```python
from build123d import *

# Parameters (mm, degrees)
SKETCH2_W               = 18
SKETCH2_H               = 43.5
BOSS_EXTRUDE1_DEPTH     = 25
CUT_EXTRUDE1_DEPTH      = 15
CUT_EXTRUDE1_DEPTH_BACK = 6.951267747
CUT_EXTRUDE2_START      = 0.4
CUT_EXTRUDE2_DEPTH      = 3.3
SKETCH5_W               = 15
SKETCH5_H               = 43.5
BOSS_EXTRUDE2_DEPTH     = 120
SKETCH6_W               = 2.2
SKETCH6_H               = 14.9
CUT_EXTRUDE3_DEPTH      = 2
CUT_EXTRUDE4_START      = -43.5
SKETCH6_3_W             = 2.2
SKETCH6_3_H             = 14.9
CUT_EXTRUDE4_DEPTH      = 2
CUT_EXTRUDE5_DEPTH      = 44.5
SKETCH8_W               = 37.1
SKETCH8_H               = 38
CUT_EXTRUDE6_DEPTH      = 16
FILLET1_R               = 10


with BuildPart() as part:
    # Sketch2 → Boss-Extrude1 (new body)
    with BuildSketch(Plane(origin=(0, 0, 0), x_dir=(1, 0, 0), z_dir=(0, 1, 0))):
        with BuildLine():
            Line((-9, 0), (-9, 21.75))
            Line((-9, 21.75), (-14.951267747, 10.950365309))
            ThreePointArc((-14.951267747, 10.950365309), (-10.583942354, 6.231534486), (-9, 0))
        make_face()
        with BuildLine():
            Line((-9, -21.75), (-9, 0))
            ThreePointArc((-9, 0), (-10.583942354, -6.231534486), (-14.951267747, -10.950365309))
            Line((-14.951267747, -10.950365309), (-9, -21.75))
        make_face()
        Rectangle(SKETCH2_W, SKETCH2_H)
    extrude(amount=BOSS_EXTRUDE1_DEPTH)

    # Sketch3 → Cut-Extrude1 (cut, two sides)
    with BuildSketch(Plane(origin=(-9, 0, 0), x_dir=(0, 0, -1), z_dir=(1, 0, 0))) as cut_extrude1_sk:
        Polygon((-5.15, 25), (5.15, 25), (7.15, 21.535898385), (-7.15, 21.535898385), align=None)
    extrude(amount=CUT_EXTRUDE1_DEPTH, mode=Mode.SUBTRACT)
    extrude(cut_extrude1_sk.sketch, amount=-CUT_EXTRUDE1_DEPTH_BACK, mode=Mode.SUBTRACT)

    # Sketch4 → Cut-Extrude2 (cut)
    with BuildSketch(Plane(origin=(-9, 0, 0), x_dir=(0, 0, -1), z_dir=(1, 0, 0)).offset(CUT_EXTRUDE2_START)):
        with BuildLine():
            Line((3.15, 29.404082691), (3.15, 4.535898385))
            ThreePointArc((3.15, 4.535898385), (0, 1.385898385), (-3.15, 4.535898385))
            Line((-3.15, 4.535898385), (-3.15, 29.404082691))
            ThreePointArc((-3.15, 29.404082691), (0, 32.554082691), (3.15, 29.404082691))
        make_face()
    extrude(amount=CUT_EXTRUDE2_DEPTH, mode=Mode.SUBTRACT)

    # Sketch5 → Boss-Extrude2 (add)
    with BuildSketch(Plane.XZ):
        with Locations((1.5, 0)):
            Rectangle(SKETCH5_W, SKETCH5_H)
    extrude(amount=BOSS_EXTRUDE2_DEPTH)

    # Sketch6 → Cut-Extrude3 (cut)
    with BuildSketch(Plane.XY.offset(21.75)):
        Polygon((-3.1, -105.1), (0.4, -105.1), (2.6, -105.1), (6.1, -105.1), (6.1, -100.9), (-3.1, -100.9), align=None)
        with Locations((1.5, -112.55)):
            Rectangle(SKETCH6_W, SKETCH6_H)
    extrude(amount=-CUT_EXTRUDE3_DEPTH, mode=Mode.SUBTRACT)

    # Sketch6<3> → Cut-Extrude4 (cut)
    with BuildSketch(Plane.XY.offset(21.75).offset(CUT_EXTRUDE4_START)):
        Polygon((-3.1, -105.1), (0.4, -105.1), (2.6, -105.1), (6.1, -105.1), (6.1, -100.9), (-3.1, -100.9), align=None)
        with Locations((1.5, -112.55)):
            Rectangle(SKETCH6_3_W, SKETCH6_3_H)
    extrude(amount=CUT_EXTRUDE4_DEPTH, mode=Mode.SUBTRACT)

    # Sketch7 → Cut-Extrude5 (cut, through all)
    with BuildSketch(Plane.XY.offset(21.75)):
        Polygon((9, -116.358920801), (3.8, -120), (9, -120), align=None)
    extrude(amount=-CUT_EXTRUDE5_DEPTH, mode=Mode.SUBTRACT)

    # Sketch8 → Cut-Extrude6 (cut, through all)
    with BuildSketch(Plane.ZY.offset(6)):
        with Locations((0, -120)):
            Rectangle(SKETCH8_W, SKETCH8_H)
    extrude(amount=-CUT_EXTRUDE6_DEPTH, mode=Mode.SUBTRACT)

    # Fillet1
    fillet1_edges = [part.edges().sort_by_distance(p)[0] for p in [
        (1.5, -101, 18.55),
        (1.5, -101, -18.55),
    ]]
    fillet(fillet1_edges, radius=FILLET1_R)


solid = part.part
```
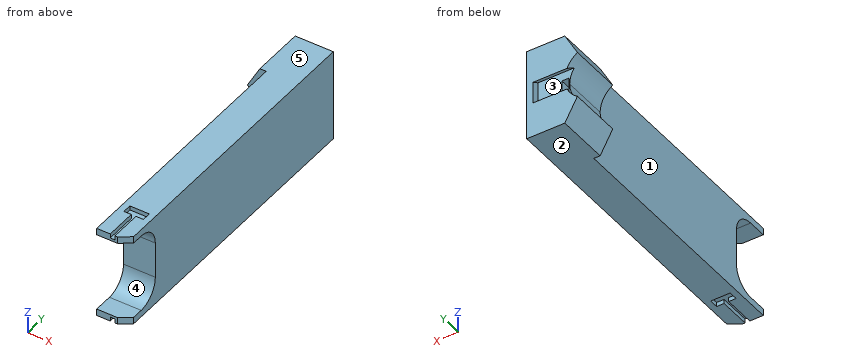
Can you work these out from the model? Positions are in its coordinate system, mm. Face numbers are marked on the shaded views. A direction names the side the tool comes from. Round coordinates to 2 decimals unless told otherwise and drop trailing zeros. Loops run counter-clockwise (first coordinate to the right, second up) from the corner with the lowest first, then second, coordinate; pieces in that order, holes last. Notation, with made-up numbers: (26, 63) -> (31, 63) arc R7 cw to (31, 67) -> close; hole circle Ø4 at (6, -38). An arc over 180 degrees is marked (long way). One line per item, written item: value. Start each with the question number.
1. For the marked faces 4 and 5, which set-ups out of +Z, -Z, +X, -X, +Y, -Y let a thin tool reach every point of the face, with its end or its side?
2. For pin 1 (22 mm diameter, centred on y = -57.5, z = -1, fed in from -X); pin 2 (4.5 mm diameter, centred on x = -9.5, z = 6, fed in from -Y); pin 3 (4 mm diameter, centred on x = 1, z = 0, fed in from -Y), each with a flat end and sliding along its axis, tell me the tip position at first contact or that it passes through.
3. If we section it at A-A, the plane y = 13.5: Write out the boundary of the cut face in (x, z), then the cut area to 3 significant figures.
4. If I drill on probe 1 along X at (y, z) = (-62.5, -9); probe 2 along Y at (x, z) = (-8.75, 10.5); probe 3 along Y at (x, z) = (3.5, 3), over which ranges is the centre line in solid material (lowest first)?
5. If we mould it in two halves opening along Z, with no side actions, what happens to the marked faces 1, 2 and 3? For each: pulls with the +Z half, pulls with the -Z half, needs draft (parallel to the pull), parting line crosses it, or undercut.
6. If we section it at B-B, the plane y = -66: Write out the boundary of the cut face in (x, z), then the cut area to 4 significant figures.
Calculated:
1. face 4: +X, -X, -Y
1. face 5: +Z, +X, -X, +Y, -Y
2. pin 1: stops at x = -6
2. pin 2: stops at y = 0
2. pin 3: stops at y = -101
3. outline: (-14.95, -10.95) -> (-9, -21.75) -> (9, -21.75) -> (9, 21.75) -> (-9, 21.75) -> (-14.95, 10.95) arc R13.05 cw to start; hole (-8.6, -3.15) -> (-5.3, -3.15) -> (-5.3, 3.15) -> (-8.6, 3.15) -> close
3. area: 865 mm²
4. probe 1: x = -6 to 9
4. probe 2: y = 0 to 25
4. probe 3: y = -101 to 21.54
5. face 1: needs draft
5. face 2: pulls with the -Z half
5. face 3: undercut
6. outline: (-6, -21.75) -> (9, -21.75) -> (9, 21.75) -> (-6, 21.75) -> close
6. area: 652.5 mm²
